Build history of the part. All positions in model axes, mm. Face numbers are marked on the shaded views. A direction names the side the tool comes from. Give positions to 0.01 mm unless a question says otherwise; leave off trailing zeros. Loops run counter-clockwise (first coordinate to the right, second up) from the corner with the lowest first, then second, coordinate; pieces in that order, holes last. Notation, with made-up numbers: (17.25, 50) -> (71.25, 50) arc R30 cw to (71.25, 87) -> close; hole circle Ø2 at (34, 18.25). An arc over 180 degrees is marked (long way). Answer as a JSON object with one key per item and string values. Group by question number.
from build123d import *

# Parameters (mm, degrees)
CHANFREIN1_SIZE = 0.4


with BuildPart() as part:
    # Esquisse1 → Révolution1 (revolve)
    with BuildSketch(Plane.XY):
        Polygon((1.6, -1.131933067), (4, -1.131933067), (4, 0.168066933), (2.47, 0.168066933), (2.47, 3.668066933), (1.6, 3.668066933), align=None)
    revolve(axis=Axis((0, 4.72147651, 0), (0, -1, 0)))

    # Chanfrein1
    chanfrein1_edges = [part.edges().sort_by_distance(p)[0] for p in [
        (-4, -1.131933067, 0),
        (-2.47, 3.668066933, 0),
    ]]
    chamfer(chanfrein1_edges, length=CHANFREIN1_SIZE)


solid = part.part
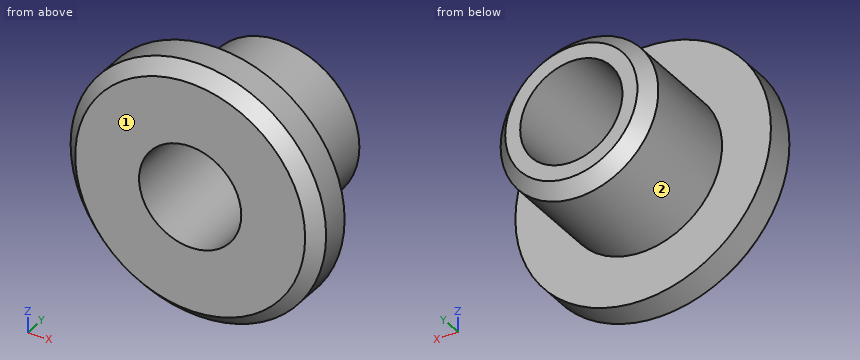
(1) Probe line 1 along Z through (x, y) = (0, -0.05); line 2 along Z through (x, y) = (0, 1.15); line 3 along Y through (x, z) = (-2.5, 1.25). List the from-to ranges inside material, lowest first. Write a range as [from, to].
(2) Saw through at D-D on y = 2.5. List the corners of the cut face in (x, z).
(3) Pin check, flat tip, straight feed: pin 1 (2 mm diameter, centred on y = 0.5, z = 0, fed in from +X). Stop position of the tip, or through.
(4) Saw through at C-C on y = 0.05. List the corners of the cut face in (x, z).
(5) 3-axis set-ups, long thin cutter, end or side, ignore diameter. For the marked faces 1 and 2: which of +Z, -Z, +X, -X, +Y, -Y reach the whole face in a straight line?
(6) Saw through at B-B on z = 0. List the corners of the cut face in (x, y), plus the area to 3 significant figures.
(7) Saw through at A-A on x = 0. List the corners of the cut face in (y, z), plus the area to 3 significant figures.
Calculated:
{
 "1": {"line 1": "z = [-4, -1.6], [1.6, 4]", "line 2": "z = [-2.47, -1.6], [1.6, 2.47]", "line 3": "y = [-1.13, 0.17]"},
 "2": {"outline": "circle Ø4.94 at (0, 0); hole circle Ø3.2 at (0, 0)"},
 "3": {"pin 1": "stops at x = 4"},
 "4": {"outline": "circle Ø8 at (0, 0); hole circle Ø3.2 at (0, 0)"},
 "5": {"face 1": "+Z, -Z, +X, -X, -Y", "face 2": "+Y"},
 "6": {"outline": "(-4, -0.73) -> (-3.6, -1.13) -> (-1.6, -1.13) -> (-1.6, 3.67) -> (-2.07, 3.67) -> (-2.47, 3.27) -> (-2.47, 0.17) -> (-4, 0.17) -> close; (1.6, -1.13) -> (3.6, -1.13) -> (4, -0.73) -> (4, 0.17) -> (2.47, 0.17) -> (2.47, 3.27) -> (2.07, 3.67) -> (1.6, 3.67) -> close", "area": "12.0 mm^2"},
 "7": {"outline": "(-1.13, -3.6) -> (-0.73, -4) -> (0.17, -4) -> (0.17, -2.47) -> (3.27, -2.47) -> (3.67, -2.07) -> (3.67, -1.6) -> (-1.13, -1.6) -> close; (-1.13, 1.6) -> (3.67, 1.6) -> (3.67, 2.07) -> (3.27, 2.47) -> (0.17, 2.47) -> (0.17, 4) -> (-0.73, 4) -> (-1.13, 3.6) -> close", "area": "12.0 mm^2"}
}
